Autodesk Inventor part; units mm, degrees
ref_plane "YZ Plane" through (0, 0, 0) normal (1, 0, 0) x (0, 1, 0)
ref_plane "XZ Plane" through (0, 0, 0) normal (0, 1, 0) x (-1, 0, 0)
ref_plane "XY Plane" through (0, 0, 0) normal (0, 0, 1) x (1, 0, 0)
sketch "Sketch2" plane through (0, 0, 0) normal (1, 0, 0) x (0, 1, 0)
  line L0 (0, 0) -> (0, -44.5)
  line L1 (17.4, -44.5) -> (17.4, 0)
  line L2 (17.4, 0) -> (25.25, 0)
  line L3 (25.25, 0) -> (25.25, -2.29)
  line L4 (24.7236, -3.0418) -> (20.366, -4.6278)
  line L5 (19.05, -6.5072) -> (19.05, -44.5)
  line L6 (19.05, -44.5) -> (17.4, -44.5)
  arc A0 (24.7236, -3.0418) -> (25.25, -2.29) centre (24.45, -2.29) ccw
  arc A1 (20.366, -4.6278) -> (19.05, -6.5072) centre (21.05, -6.5072) ccw
  dimension "OD" = 38.1
  dimension "THW" = 1.65
  dimension "L" = 44.5
  dimension "d3" = 50.5
  dimension "d4" = 0.8
  dimension "d5" = 2.29
  dimension "d6" = 2
  dimension "d7" = 20
revolve "Revolution1" add sketch "Sketch2" angle 360 about axis through (0, 0, 0) along (0, 0, -1)
properties part number "Ferrule-38.1" material "Stainless Steel, 316L"
Source: CAD feature listing. Evaluate the final solid. Frame: model axes, mm. Coordinates: 2 decimals unless noted, no trailing zeros. Write each loop counter-clockwise with the first axis right and the second up, starting at its lowest first coordinate (ties: lowest second). Pieces come first, ordered by that corner, then holes. Notation, with made-up numbers: (-30.75, 28.5) -> (5.25, 28.5) arc R30 cw to (5.25, 60.5) -> close; hole circle Ø5 at (-39, 9). An arc over 180 degrees is marked (long way). Return JSON: item names as keys, results as strings. Group by question number.
1) Contact query for flat-ended pins moving along their axis: P1, Ø3, axis at y = 10, z = -10.5, coming from the -X side; P2, Ø8, axis at y = -12, z = -21, coming from the -X side; P3, Ø4, axis at x = -19, z = -19, coming from the -Y side. Output: stop coordinate, or through.
2) Section query A-A, the plane x = 0. Return loops of the section in (y, z).
3) Ray query, line 1 along X through (y, z) = (0, -22); line 2 along Y through (x, z) = (15.5, -36). Return the intervals inside material, ascending.
4) Section query C-C, the plane z = -25.5. Return loops of the section in (x, y).
5) Mould query, pull axis X, two halves, no side actions, for faces 1 (the face through (-16.5, -6, 0)), 2 (the face through (16.986, -3.772, -21.938)), 3 (the face through (-11.59, -15.12, -25.77)). Classes: +X half, -X half, draft (parallel to the pull), parting line (faces both ways), or undercut.
From the geometry:
{
 "1": {"P1": "x = -17.05", "P2": "x = -17.29", "P3": "y = -8.6"},
 "2": {"outline": "(-25.25, -2.29) arc R0.8 ccw to (-24.72, -3.04) -> (-20.37, -4.63) arc R2 cw to (-19.05, -6.51) -> (-19.05, -44.5) -> (-17.4, -44.5) -> (-17.4, 0) -> (-25.25, 0) -> close; (17.4, -44.5) -> (19.05, -44.5) -> (19.05, -6.51) arc R2 cw to (20.37, -4.63) -> (24.72, -3.04) arc R0.8 ccw to (25.25, -2.29) -> (25.25, 0) -> (17.4, 0) -> close"},
 "3": {"line 1": "-19.05 to -17.4, 17.4 to 19.05", "line 2": "-11.07 to -7.91, 7.91 to 11.07"},
 "4": {"outline": "circle Ø38.1 at (0, 0); hole circle Ø34.8 at (0, 0)"},
 "5": {"face 1": "draft", "face 2": "undercut", "face 3": "parting line"}
}
